Part model, mm, in its own coordinate system. A direction names the side the tool comes from. Give positions to 0.01 mm unless a question says otherwise; leave off trailing zeros. Order: outer loops, then holes, each group sorted by start corner. A loop starts at its lowest first (then second) coordinate and runs counter-clockwise, first axis right, second up. Notation, with made-up numbers: (35, 37.25) -> (43, 37.25) arc R38 ccw to (43, 75.25) -> close; hole circle Ø4 at (-0.5, 15.25). An arc over 180 degrees is marked (long way). Write item = value, one per line. Start each with the question number.
Item 1: Tool access for faces 1 (the face through (23.876, -76, 7)), 2 (the face through (0, -7, 7)): list every direction of +Z, -Z, +X, -X, +Y, -Y with a clear straight run to the whole face (end or side of a thin tool).
Item 2: Band-saw the part on A-A on z = -416.5. Write the cut outline in (x, y), plus the area to 3 significant figures.
Item 3: Band-saw the part on B-B on y = -36. Write the cut outline in (x, z).
Item 4: Drill centre lines: line 1 along Y through (x, z) = (27, 482.5); line 2 along Y through (x, z) = (22, -230); line 3 along X through (y, z) = (-9, 166.5). Where is each one in solid material? Low to high.
Item 5: Pull direction Y, two halves, no side cores. Call faces 3 (the face through (15, -533.4, -7)), 4 (the face through (14.351, -1, 7)), 5 (the face through (15, 533.4, -7)), 6 (the face through (12, -7, -527.05)): +Y half, -Y half, draft (parallel to the pull), parting line (faces both ways), or undercut.
Item 6: Flat gauge pin, fed straight in: P1, Ø20.5, axis at y = -76, z = 95.5, coming from the +X side. Where does the tip first touch, or does it go through?
```python
from build123d import *

# Parameters (mm, degrees)
F0_W     = 1066.8
F0_H     = 1054.1
F1_DEPTH = 30.226
F2_W     = 177.8
F2_H     = 1054.1
F3_DEPTH = 6.35
F4_W     = 127
F4_H     = 1054.1
F5_DEPTH = 9.525


with BuildPart() as f1:
    # F0 (on Right) → F1 (new body)
    with BuildSketch(Plane.YZ):
        Rectangle(F0_W, F0_H)
    extrude(amount=F1_DEPTH)

    # F2 (on face) → F3 (cut)
    with BuildSketch(Plane.YZ.offset(30.226)):
        Rectangle(F2_W, F2_H)
    extrude(amount=-F3_DEPTH, mode=Mode.SUBTRACT)

    # F4 (on face) → F5 (cut)
    with BuildSketch(Plane.YZ.offset(23.876)):
        Rectangle(F4_W, F4_H)
    extrude(amount=-F5_DEPTH, mode=Mode.SUBTRACT)


solid = f1.part
```
Values found:
q1.face_1 = +Z, -Z, +X
q1.face_2 = +Z, -Z, -X, +Y, -Y
q2.outline = (0, -533.4) -> (30.23, -533.4) -> (30.23, -88.9) -> (23.88, -88.9) -> (23.88, -63.5) -> (14.35, -63.5) -> (14.35, 63.5) -> (23.88, 63.5) -> (23.88, 88.9) -> (30.23, 88.9) -> (30.23, 533.4) -> (0, 533.4) -> close
q2.area = 29,900 mm^2
q3.outline = (0, -527.05) -> (14.35, -527.05) -> (14.35, 527.05) -> (0, 527.05) -> close
q4.line_1 = -533.4 to -88.9, 88.9 to 533.4
q4.line_2 = -533.4 to -63.5, 63.5 to 533.4
q4.line_3 = 0 to 14.35
q5.face_3 = -Y half
q5.face_4 = undercut
q5.face_5 = +Y half
q5.face_6 = draft
q6.P1 = 23.88
